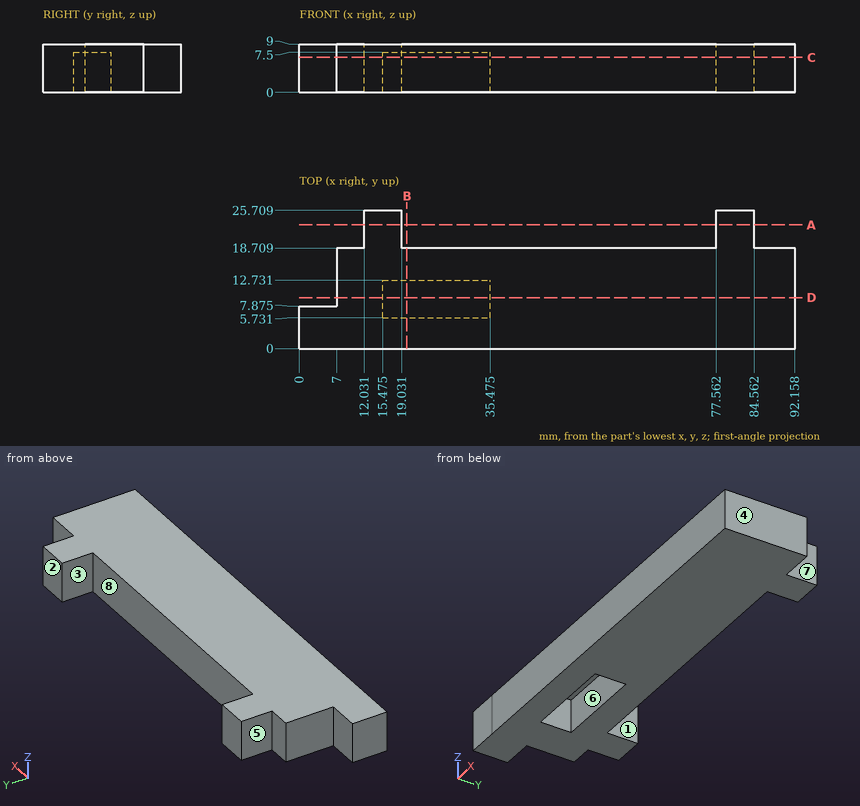
For this review, use the dimensioned drawing (mm, ordinates from the lowest corner) and the shaded views. A direction names the side the tool comes from. Round coordinates to 2 decimals unless told otherwise and drop trailing zeros. Order: outer loops, then holes, each group sorted by start corner. A loop starts at its lowest first (then second) coordinate and runs counter-clockwise, first axis right, second up.
1) Consider section A-A (y = 23). State the section outline as (x, z) points.
The answers:
outline: (12.03, 0) - (19.03, 0) - (19.03, 9) - (12.03, 9) - close; (77.56, 0) - (84.56, 0) - (84.56, 9) - (77.56, 9) - close
2) Clearance check with flat-ended pins moving along their axes: pin 1 Ø3.5 at (y, z) = (20.5, 3.5) entering from -X; pin 2 Ø1 at (x, y) = (30.5, 7) entering from -Z; pin 3 Ø1 at (x, z) = (49.5, 8) entering from +Y. State where each tip first meets the part, or that it passes through.
The answers:
pin 1: stops at x = 12.03
pin 2: stops at z = 7.5
pin 3: stops at y = 18.71
3) Draft analysis for pull direction X (two halves, no side actions). For the marked faces 1, 2, 3 and 4, state which applies: released by +X, released by -X, zero draft, split by the parting line, or undercut.
The answers:
face 1: undercut
face 2: zero draft
face 3: undercut
face 4: released by +X
4) Consider section B-B (x = 20). State the section outline as (y, z) points, plus the area to 3 significant figures.
The answers:
outline: (0, 0) - (5.73, 0) - (5.73, 7.5) - (12.73, 7.5) - (12.73, 0) - (18.71, 0) - (18.71, 9) - (0, 9) - close
area: 116 mm2
5) Consider section D-D (y = 9.5). State the section outline as (x, z) points (1 decimal).
The answers:
outline: (7, 0) - (15.5, 0) - (15.5, 7.5) - (35.5, 7.5) - (35.5, 0) - (92.2, 0) - (92.2, 9) - (7, 9) - close
6) For L1, parallel to X at y = 18.75, z = 8; L2, parallel to Y at x = 34, z = 4; L3, parallel to X at y = 6, z = 3.75 (1 decimal), list the stretches that pass through material, from the lowest coordinate up.
The answers:
L1: x = 12.03 to 19.03, 77.56 to 84.56
L2: y = 0 to 5.73, 12.73 to 18.71
L3: x = 0 to 15.5, 35.5 to 92.2
7) Consider section C-C (z = 6.5). State the section outline as (x, y) points (1 decimal), plus the area to 3 significant figures.
The answers:
outline: (0, 0) - (92.2, 0) - (92.2, 18.7) - (84.6, 18.7) - (84.6, 25.7) - (77.6, 25.7) - (77.6, 18.7) - (19, 18.7) - (19, 25.7) - (12, 25.7) - (12, 18.7) - (7, 18.7) - (7, 7.9) - (0, 7.9) - close; hole (15.5, 5.7) - (35.5, 5.7) - (35.5, 12.7) - (15.5, 12.7) - close
area: 1,610 mm2
8) Machinability: for the marked faces 5, 6, 7 and 8, which of the approach directions +Z, -Z, +X, -X, +Y, -Y give a long, thin tool a straight path to every point of the face, cutting with its end or side? Answer none if there is none.
The answers:
face 5: +Z, -Z, -X, +Y
face 6: -Z
face 7: +Z, -Z, +X, +Y
face 8: +Z, -Z, +Y
